from build123d import *

# Parameters (mm, degrees)
SKETCH_2_W          = 18
SKETCH_2_H          = 21.5
EXTRUDE_1_DEPTH     = 4
SKETCH_3_W          = 12
SKETCH_3_H          = 17.5
CUT_EXTRUDE_1_DEPTH = 29.324018077
FILLET_1_R          = 5
FILLET_2_R          = 5
SKETCH_4_W          = 4
SKETCH_4_H          = 2
CUT_EXTRUDE_2_DEPTH = 29.324018077
SKETCH_5_W          = 4
SKETCH_5_H          = 3
EXTRUDE_2_DEPTH     = 0.2
CUT_EXTRUDE_3_DEPTH = 29.324018077


with BuildPart() as part:
    # ｽｹｯﾁ2 → ﾎﾞｽ - 押し出し1 (new body)
    with BuildSketch(Plane.XY):
        with Locations((9, 10.75)):
            Rectangle(SKETCH_2_W, SKETCH_2_H)
    extrude(amount=EXTRUDE_1_DEPTH)

    # ｽｹｯﾁ3 → ｶｯﾄ - 押し出し1 (cut, through all)
    with BuildSketch(Plane.XY.offset(4)):
        with Locations((9, 8.75)):
            Rectangle(SKETCH_3_W, SKETCH_3_H)
    extrude(amount=-CUT_EXTRUDE_1_DEPTH, mode=Mode.SUBTRACT)

    # ﾌｨﾚｯﾄ1
    fillet_1_edges = [part.edges().sort_by_distance(p)[0] for p in [
        (3, 17.5, 2),
        (15, 17.5, 2),
    ]]
    fillet(fillet_1_edges, radius=FILLET_1_R)

    # ﾌｨﾚｯﾄ2
    fillet_2_edges = [part.edges().sort_by_distance(p)[0] for p in [
        (0, 21.5, 2),
        (18, 21.5, 2),
    ]]
    fillet(fillet_2_edges, radius=FILLET_2_R)

    # ｽｹｯﾁ4 → ｶｯﾄ - 押し出し2 (cut, through all)
    with BuildSketch(Plane.XY.offset(4)):
        with Locations((9, 19.400947982)):
            Rectangle(SKETCH_4_W, SKETCH_4_H)
    extrude(amount=-CUT_EXTRUDE_2_DEPTH, mode=Mode.SUBTRACT)

    # ｽｹｯﾁ5 → ﾎﾞｽ - 押し出し2 (add)
    with BuildSketch(Plane.ZY):
        with Locations((2, 2.5)):
            Rectangle(SKETCH_5_W, SKETCH_5_H)
    extrude(amount=EXTRUDE_2_DEPTH)

    # ｽｹｯﾁ6 → ｶｯﾄ - 押し出し3 (cut, through all)
    with BuildSketch(Plane.XY.offset(4)):
        Polygon((0, 1), (-0.2, 2.5), (-0.2, 1), align=None)
    extrude(amount=-CUT_EXTRUDE_3_DEPTH, mode=Mode.SUBTRACT)


solid = part.part
Could you check a few things on this model? Use its own coordinates, in mm. A direction names the side the tool comes from. Give positions to 0.01 mm unless a question says otherwise; leave off trailing zeros. Order: outer loops, then holes, each group sorted by start corner. A loop starts at its lowest first (then second) coordinate and runs counter-clockwise, first axis right, second up.
1. Suppose I cut it at D-D (x = 16). Write out the boundary of the cut face in (y, z), plus the area to 3 significant figures.
Answers below:
outline: (0, 0) - (20.5, 0) - (20.5, 4) - (0, 4) - close
area: 82.0 mm2
2. I need wall thicknesses on L1, parallel to X at y = 11, z = 3.3; L2, parallel to X at y = 16.75, z = 0.75; L3, parallel to Y at x = 13, z = 1.6. Which ranges of each line are inside material? Lowest first, please.
Answers below:
L1: x = 0 to 3, 15 to 18
L2: x = 0.01 to 5.37, 12.63 to 17.99
L3: y = 16.5 to 21.5
3. Which directions (+Z, -Z, +X, -X, +Y, -Y) give clear straight access to the entire face, cutting with the end or side of a thin tool? Please do faces 4 (the flat face through (11, 19, 2)), 5 (the flat face through (0, 0.5, 2)), 6 (the flat face through (0, 10, 2)).
Answers below:
face 4: +Z, -Z
face 5: +Z, -Z, -X, -Y
face 6: +Z, -Z, -X, +Y
4. For pin 1 (0.8 mm diameter, centred on y = 0.5, z = 1.5, fed in from -X); pin 2 (2 mm diameter, centred on y = 19, z = 2.5, fed in from -X); pin 3 (1.2 mm diameter, centred on x = 9.5, z = 2, fed in from -Y), each with a flat end and sliding along its axis, tell me the tip position at first contact or that it passes through.
Answers below:
pin 1: stops at x = 0
pin 2: stops at x = 0.23
pin 3: stops at y = 17.5
5. Suppose I cut it at B-B (z = 1.35). Write out the boundary of the cut face in (x, y).
Answers below:
outline: (-0.2, 2.5) - (0, 1) - (0, 0) - (3, 0) - (3, 12.5) arc R5 cw to (8, 17.5) - (10, 17.5) arc R5 cw to (15, 12.5) - (15, 0) - (18, 0) - (18, 16.5) arc R5 ccw to (13, 21.5) - (5, 21.5) arc R5 ccw to (0, 16.5) - (0, 4) - (-0.2, 4) - close; hole (7, 18.4) - (11, 18.4) - (11, 20.4) - (7, 20.4) - close
6. Suppose I cut it at C-C (x = 8.75). Write out the boundary of the cut face in (y, z).
Answers below:
outline: (17.5, 0) - (18.4, 0) - (18.4, 4) - (17.5, 4) - close; (20.4, 0) - (21.5, 0) - (21.5, 4) - (20.4, 4) - close
7. Thinking about a two-plate mould opening in Y: for faces 1 (the flat face through (9, 17.5, 2)), 2 (the flat face through (7, 19, 2)), 3 (the flat face through (9, 18, 4)), which applies, +Y half, -Y half, draft (parallel to the pull), parting line (faces both ways), or undercut?
Answers below:
face 1: -Y half
face 2: undercut
face 3: draft
8. Suppose I cut it at A-A (y = 3.5). Write out the boundary of the cut face in (x, z), plus the area to 3 significant figures.
Answers below:
outline: (-0.2, 0) - (3, 0) - (3, 4) - (-0.2, 4) - close; (15, 0) - (18, 0) - (18, 4) - (15, 4) - close
area: 24.8 mm2
